Study the drawing (mm; zero at the part's minimum x, y, z) and answer. Coordinates: 2 decimals unless noted, no trailing zeros. Answer as CSV lines item,"result".
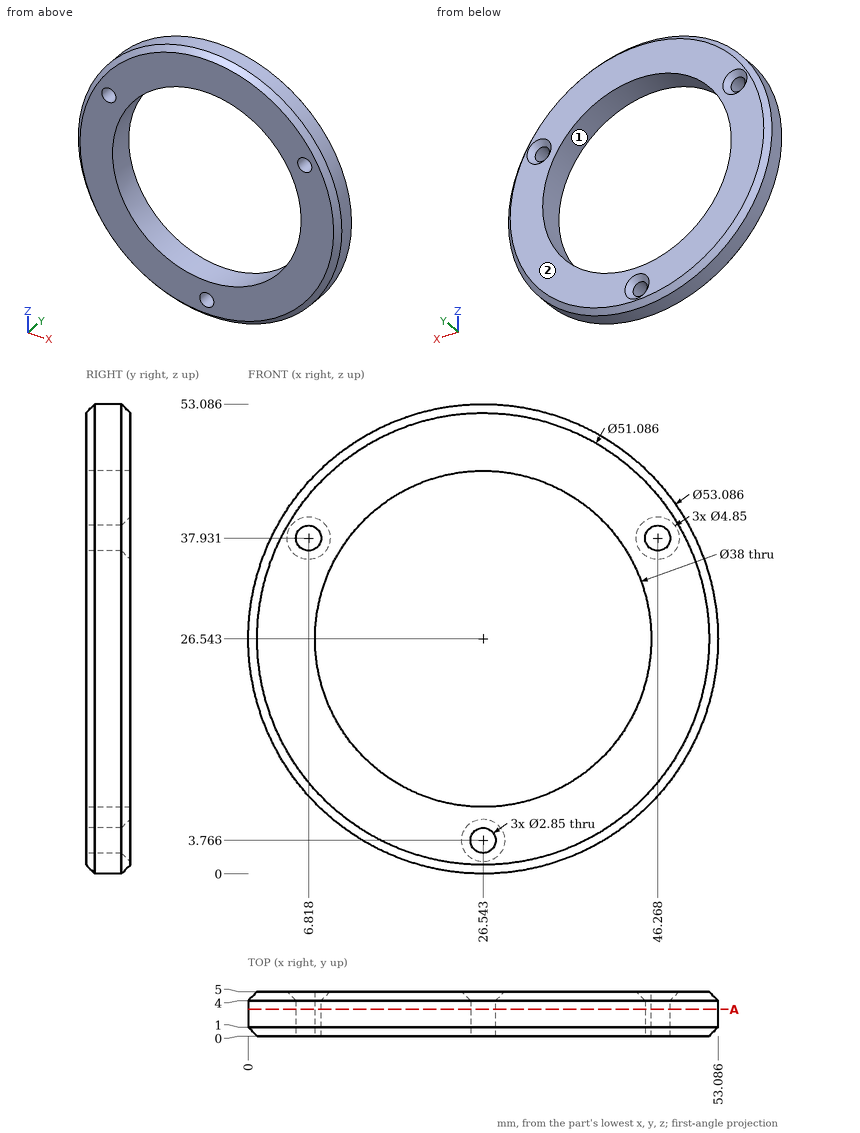
Q1. For a pull along X with two mould halves and no side action, classify the marked faces 1 and 2 as pulls with the +X half, pulls with the -X half, needs draft (parallel to the pull), parting line crosses it, or undercut.
Results:
face 1,"undercut"
face 2,"needs draft"
Q2. Find the intervals of material crossed by probe 1 along X at (y, z) = (4.2, 38) (1 decimal); probe 2 along X at (y, z) = (0.85, 32) (1 decimal); probe 3 along Z at (x, y) = (17, 1.95) (1 decimal), in increasing order. Write a range as [from, to].
Results:
probe 1,"x = [2.8, 5.2], [8.4, 11.4], [41.7, 44.6], [47.9, 50.3]"
probe 2,"x = [0.7, 8.3], [44.7, 52.4]"
probe 3,"z = [1.8, 10.1], [43, 51.3]"
Q3. Given pin 1 Ø1 at (y, z) = (1.5, 38.5) entering from -X; pin 2 Ø8 at (x, z) = (44, 37.5) entering from +Y; pin 3 Ø1.5 at (y, z) = (1.5, 17.5) entering from +X; pin 4 Ø4.5 at (x, z) = (46.27, 37.93) entering from +Y, each flat-ended and moving along its own axis, determine where each tip first touches the part or whether it passes through.
Results:
pin 1,"stops at x = 2.6"
pin 2,"stops at y = 5"
pin 3,"stops at x = 51.76"
pin 4,"stops at y = 4.83"
Q4. A cutting plane is placed at A-A, the plane y = 3. Give the number of separate pieces and of enclosed holes in the cut face, and give its area (3 significant figures).
Results:
separate pieces,"1"
enclosed holes,"4"
area,"1,060 mm²"
